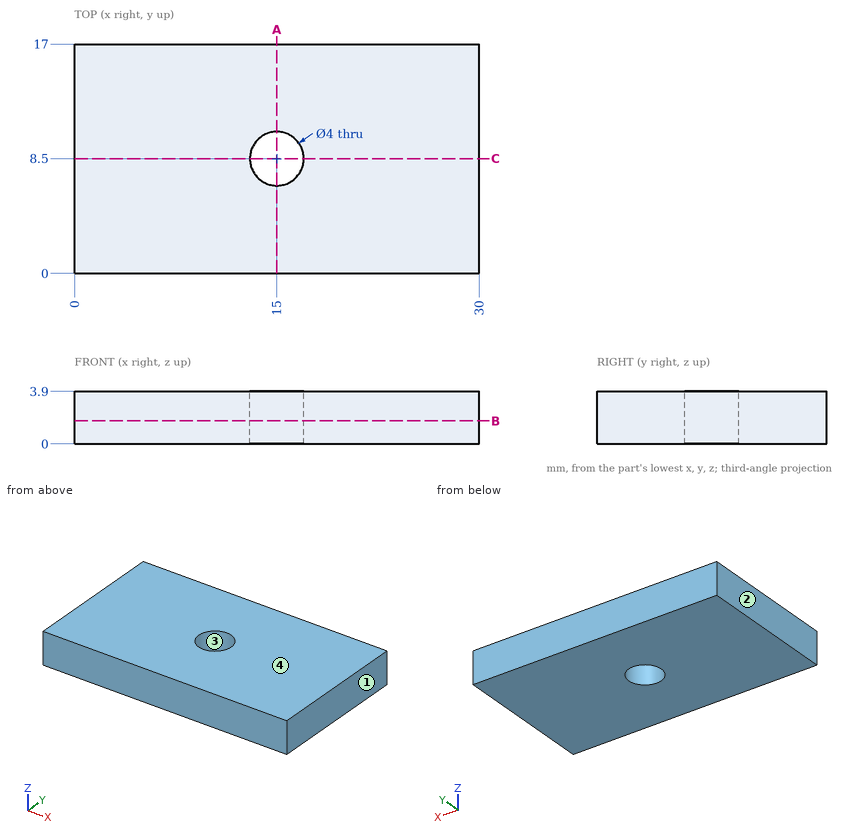
Design review of the part shown in the three views and the two pictorial views. Dimensions are in mm from the part's minimum x, y and z. Round coordinates to 2 decimals unless told otherwise and drop trailing zeros. Order: outer loops, then holes, each group sorted by start corner. A loop starts at its lowest first (then second) coordinate and runs counter-clockwise, first axis right, second up.
(1) Wall thickness on L1, parallel to Y at x = 15, z = 1.8; L2, parallel to X at y = 8, z = 0.4: over which ranges is each line inside the solid? List them lowest first.
Working result:
L1: y = 0 to 6.5, 10.5 to 17
L2: x = 0 to 13.06, 16.94 to 30
(2) Mouldability with a two-part tool opening along X and no side actions: class the marked faces 1, 2, 3 and 4 as released by +X, released by -X, zero draft, split by the parting line, or undercut.
Working result:
face 1: released by +X
face 2: released by -X
face 3: undercut
face 4: zero draft
(3) Take a section at C-C, the plane y = 8.5. State the section outline as (x, z) points.
Working result:
outline: (0, 0) - (13, 0) - (13, 3.9) - (0, 3.9) - close; (17, 0) - (30, 0) - (30, 3.9) - (17, 3.9) - close
(4) Take a section at A-A, the plane x = 15. State the section outline as (y, z) points, plus the area to 3 significant figures.
Working result:
outline: (0, 0) - (6.5, 0) - (6.5, 3.9) - (0, 3.9) - close; (10.5, 0) - (17, 0) - (17, 3.9) - (10.5, 3.9) - close
area: 50.7 mm2
(5) Take a section at B-B, the plane z = 1.7. State the section outline as (x, y) points.
Working result:
outline: (0, 0) - (30, 0) - (30, 17) - (0, 17) - close; hole circle Ø4 at (15, 8.5)
(6) For P1, Ø10, axis at x = 19, y = 7.5, coming from the -Z side, flat-tipped, find the tip position at first contact; note if it passes through.
Working result:
P1: stops at z = 0
